```python
from build123d import *

# Parameters (mm, degrees)
SKETCH_1_W          = 157
SKETCH_1_H          = 345
EXTRUDE_1_DEPTH     = 4.5
CUT_EXTRUDE_1_DEPTH = 4.5
SKETCH_3_R          = 2.6
SKETCH_3_R_2        = 1.6
CUT_EXTRUDE_2_DEPTH = 4.5
FILLET_1_R          = 5


with BuildPart() as part:
    # 草图1 → 凸台-拉伸1 (new body)
    with BuildSketch(Plane.XY):
        with Locations((78.5, 172.5)):
            Rectangle(SKETCH_1_W, SKETCH_1_H)
    extrude(amount=EXTRUDE_1_DEPTH)

    # 草图2 → 切除-拉伸1 (cut)
    with BuildSketch(Plane.XY.offset(4.5)):
        with BuildLine():
            Line((20, 60), (65, 60))
            ThreePointArc((65, 60), (72.071067812, 57.071067812), (75, 50))
            Line((75, 50), (75, 20))
            ThreePointArc((75, 20), (72.071067812, 12.928932188), (65, 10))
            Line((65, 10), (20, 10))
            ThreePointArc((20, 10), (12.928932188, 12.928932188), (10, 20))
            Line((10, 20), (10, 50))
            ThreePointArc((10, 50), (12.928932188, 57.071067812), (20, 60))
        make_face()
        with BuildLine():
            Line((92, 60), (137, 60))
            ThreePointArc((137, 60), (144.071067812, 57.071067812), (147, 50))
            Line((147, 50), (147, 20))
            ThreePointArc((147, 20), (144.071067812, 12.928932188), (137, 10))
            Line((137, 10), (92, 10))
            ThreePointArc((92, 10), (84.928932188, 12.928932188), (82, 20))
            Line((82, 20), (82, 50))
            ThreePointArc((82, 50), (84.928932188, 57.071067812), (92, 60))
        make_face()
        with BuildLine():
            Line((92, 170), (137, 170))
            ThreePointArc((137, 170), (144.071067812, 167.071067812), (147, 160))
            Line((147, 160), (147, 130))
            ThreePointArc((147, 130), (144.071067812, 122.928932188), (137, 120))
            Line((137, 120), (92, 120))
            ThreePointArc((92, 120), (84.928932188, 122.928932188), (82, 130))
            Line((82, 130), (82, 160))
            ThreePointArc((82, 160), (84.928932188, 167.071067812), (92, 170))
        make_face()
        with BuildLine():
            Line((92, 280), (137, 280))
            ThreePointArc((137, 280), (144.071067812, 277.071067812), (147, 270))
            Line((147, 270), (147, 240))
            ThreePointArc((147, 240), (144.071067812, 232.928932188), (137, 230))
            Line((137, 230), (92, 230))
            ThreePointArc((92, 230), (84.928932188, 232.928932188), (82, 240))
            Line((82, 240), (82, 270))
            ThreePointArc((82, 270), (84.928932188, 277.071067812), (92, 280))
        make_face()
        with BuildLine():
            Line((20, 170), (65, 170))
            ThreePointArc((65, 170), (72.071067812, 167.071067812), (75, 160))
            Line((75, 160), (75, 130))
            ThreePointArc((75, 130), (72.071067812, 122.928932188), (65, 120))
            Line((65, 120), (20, 120))
            ThreePointArc((20, 120), (12.928932188, 122.928932188), (10, 130))
            Line((10, 130), (10, 160))
            ThreePointArc((10, 160), (12.928932188, 167.071067812), (20, 170))
        make_face()
        with BuildLine():
            Line((20, 280), (65, 280))
            ThreePointArc((65, 280), (72.071067812, 277.071067812), (75, 270))
            Line((75, 270), (75, 240))
            ThreePointArc((75, 240), (72.071067812, 232.928932188), (65, 230))
            Line((65, 230), (20, 230))
            ThreePointArc((20, 230), (12.928932188, 232.928932188), (10, 240))
            Line((10, 240), (10, 270))
            ThreePointArc((10, 270), (12.928932188, 277.071067812), (20, 280))
        make_face()
    extrude(amount=-CUT_EXTRUDE_1_DEPTH, mode=Mode.SUBTRACT)

    # 草图3 → 切除-拉伸2 (cut)
    with BuildSketch(Plane.XY.offset(4.5)):
        with Locations((7, 338)):
            Circle(SKETCH_3_R)
        with Locations((150, 338)):
            Circle(SKETCH_3_R)
        with Locations((150, 7)):
            Circle(SKETCH_3_R)
        with Locations((7, 7)):
            Circle(SKETCH_3_R)
        with Locations((150, 172.5)):
            Circle(SKETCH_3_R)
        with Locations((7, 172.5)):
            Circle(SKETCH_3_R)
        with Locations((78.5, 172.5)):
            Circle(SKETCH_3_R_2)
        with Locations((78.5, 227.5)):
            Circle(SKETCH_3_R)
        with Locations((78.5, 117.5)):
            Circle(SKETCH_3_R)
    extrude(amount=-CUT_EXTRUDE_2_DEPTH, mode=Mode.SUBTRACT)

    # 圆角1
    fillet_1_edges = [part.edges().sort_by_distance(p)[0] for p in [
        (0, 345, 2.25),
        (157, 345, 2.25),
        (157, 0, 2.25),
        (0, 0, 2.25),
    ]]
    fillet(fillet_1_edges, radius=FILLET_1_R)


solid = part.part
```
For this review, take the finished solid that the model builds, in its own axes (mm). A direction names the side the tool comes from. Round coordinates to 2 decimals unless told otherwise and drop trailing zeros. Write each loop counter-clockwise with the first axis right and the second up, starting at its lowest first coordinate (ties: lowest second). Pieces come first, ordered by that corner, then holes. Notation, with made-up numbers: (84.5, 4.5) - (115.5, 4.5) arc R17 ccw to (115.5, 25.5) - close; hole circle Ø3 at (1, 48.25). An arc over 180 degrees is marked (long way). Use CSV: the item, a comma, the result in double quotes.
1) The part is to be moulded in two halves that separate along Y. For faces 3 (the flat face through (77, 213, 4.5)), 4 (the cylindrical face through (85.01, 122.85, 2.28)), say which applies: pulls with the +Y half, pulls with the -Y half, needs draft (parallel to the pull), parting line crosses it, or undercut.
Conclusion:
face 3,"needs draft"
face 4,"undercut"
2) Clearance check with a flat-ended pin moving along its axis: pin 1 Ø4.5 at (x, y) = (150, 338) entering from -Z. State where the tip first meets the part, or that it passes through.
Conclusion:
pin 1,"passes through"
3) Add section B-B on x = 24. Write out the cut boundary in (y, z).
Conclusion:
outline,"(0, 0) - (10, 0) - (10, 4.5) - (0, 4.5) - close; (60, 0) - (120, 0) - (120, 4.5) - (60, 4.5) - close; (170, 0) - (230, 0) - (230, 4.5) - (170, 4.5) - close; (280, 0) - (345, 0) - (345, 4.5) - (280, 4.5) - close"
4) Add section C-C on z = 1.35. Count the separate pieces of the cut face and the enclosed holes in it, and give its area (3 significant figures).
Conclusion:
separate pieces,"1"
enclosed holes,"15"
area,"35,000 mm^2"
5) Wall thickness on line 1 along Y through (x, z) = (7, 3.25); line 2 along Y through (x, z) = (62, 0.85); line 3 along X through (y, z) = (270.5, 1.6): over which ranges is each line inside the solid? List them lowest first. Write a range as from..to.
Conclusion:
line 1,"y = 0..4.4, 9.6..169.9, 175.1..335.4, 340.6..345"
line 2,"y = 0..10, 60..120, 170..230, 280..345"
line 3,"x = 0..10.01, 74.99..82.01, 146.99..157"
6) For faces 1 (the cylindrical face through (12.85, 166.99, 2.28)), 2 (the flat face through (77, 213, 0)), list the 3-axis set-ups (+Z, -Z, +X, -X, +Y, -Y) from which the entire face can be reached by the end or side of a thin tool; tool diameter is ignored.
Conclusion:
face 1,"+Z, -Z"
face 2,"-Z, +X, -X, +Y, -Y"
7) Add section A-A on y = 27.5. Write out the cut boundary in (x, z).
Conclusion:
outline,"(0, 0) - (10, 0) - (10, 4.5) - (0, 4.5) - close; (75, 0) - (82, 0) - (82, 4.5) - (75, 4.5) - close; (147, 0) - (157, 0) - (157, 4.5) - (147, 4.5) - close"
